Geometry: final body of the model. Coordinates: model frame, mm. A direction names the side the tool comes from. Coordinates: 2 decimals unless noted, no trailing zeros. Write each loop counter-clockwise with the first axis right and the second up, starting at its lowest first coordinate (ties: lowest second). Pieces come first, ordered by that corner, then holes. Notation, with made-up numbers: (63.5, 14) -> (105.5, 14) arc R15 cw to (105.5, 29) -> close; hole circle Ø9 at (71, -33). An arc over 180 degrees is marked (long way). One line per item, written item: value.
```python
from build123d import *

# Parameters (mm, degrees)
SCHIZZO2_R                   = 5.1
SCHIZZO2_R_2                 = 3.5
ESTRUSIONE_ESTRUSIONE1_DEPTH = 8
SCHIZZO4_R                   = 11
TAGLIO_ESTRUSIONE1_DEPTH     = 3.7
SCHIZZO5_R                   = 1.1
TAGLIO_ESTRUSIONE2_DEPTH     = 3


with BuildPart() as part:
    # Schizzo2 → Estrusione-Estrusione1 (new body)
    with BuildSketch(Plane(origin=(0, 0, 0), x_dir=(1, 0, 0), z_dir=(0, 1, 0))):
        with BuildLine():
            Line((70, -15), (-70, -15))
            ThreePointArc((-70, -15), (-85, 0), (-70, 15))
            Line((-70, 15), (70, 15))
            ThreePointArc((70, 15), (85, 0), (70, -15))
        make_face()
        with Locations(Location((70, 0, 0), (0, 0, 270))):
            Circle(SCHIZZO2_R, mode=Mode.SUBTRACT)
        with Locations(Location((-70, 0, 0), (0, 0, 270))):
            Circle(SCHIZZO2_R_2, mode=Mode.SUBTRACT)
    extrude(amount=ESTRUSIONE_ESTRUSIONE1_DEPTH)

    # Schizzo4 → Taglio-Estrusione1 (cut)
    with BuildSketch(Plane.XZ):
        with Locations(Location((-70, 0, 0), (0, 0, 270))):
            Circle(SCHIZZO4_R)
    extrude(amount=-TAGLIO_ESTRUSIONE1_DEPTH, mode=Mode.SUBTRACT)

    # Schizzo5 → Taglio-Estrusione2 (cut)
    with BuildSketch(Plane.XZ.offset(-3.7)):
        with Locations(Location((-75.66, 5.66, 0), (0, 0, 270))):
            Circle(SCHIZZO5_R)
        with Locations(Location((-64.34, 5.66, 0), (0, 0, 90))):
            Circle(SCHIZZO5_R)
        with Locations(Location((-64.34, -5.66, 0), (0, 0, 270))):
            Circle(SCHIZZO5_R)
        with Locations(Location((-75.66, -5.66, 0), (0, 0, 90))):
            Circle(SCHIZZO5_R)
    extrude(amount=-TAGLIO_ESTRUSIONE2_DEPTH, mode=Mode.SUBTRACT)


solid = part.part
```
(1) Section D-D (z = 8.5). Return the cut outline in (x, y), then the cut area to 3 significant figures.
Responses:
outline: (-82.36, 0) -> (-76.98, 0) -> (-76.98, 3.7) -> (-63.02, 3.7) -> (-63.02, 0) -> (82.36, 0) -> (82.36, 8) -> (-82.36, 8) -> close
area: 1,270 mm2
(2) Line query: line 1 (X direction, y = 4.7, z = 0); line 2 (Z direction, x = -64.34, y = 4.4); line 3 (X direction, y = 4.75, z = 5.66). Output: solid intervals per line, ascending. Write a range as [from, to].
Responses:
line 1: x = [-85, -73.5], [-66.5, 64.9], [75.1, 85]
line 2: z = [-15, -6.76], [-4.56, 4.56], [6.76, 15]
line 3: x = [-83.89, -76.76], [-74.56, -65.44], [-63.24, 83.89]
(3) Pull-direction query (Z, two-part tool) for faces 3 (the cylindrical face through (-59.094, 1.824, 1.432)), 4 (the flat face through (1, 4, 15)), 5 (the flat face through (1, 0, 0)); classes: released by +Z, released by -Z, zero draft, split by the parting line, or undercut.
Responses:
face 3: undercut
face 4: released by +Z
face 5: zero draft
(4) Section A-A (x = 72). Return the cut outline in (y, z).
Responses:
outline: (0, -14.87) -> (8, -14.87) -> (8, -4.69) -> (0, -4.69) -> close; (0, 4.69) -> (8, 4.69) -> (8, 14.87) -> (0, 14.87) -> close
(5) Reachability of faces 1 (the cylindrical face through (75, 4, -1)), 2 (the flat face through (-67, 3.7, 3)) from +Z, -Z, +X, -X, +Y, -Y: full face, straight path, thin tool, end or side. Return the list, or none.
Responses:
face 1: +Y, -Y
face 2: -Y
(6) First-contact query: pin 1 (17.5 mm diameter, centred on x = -70, z = 0, fed in from -Y); pin 2 (11 mm diameter, centred on x = -70, z = 0, fed in from +Y); pin 3 (1.3 mm diameter, centred on x = -64.34, z = -5.66, fed in from -Y); pin 4 (9 mm diameter, centred on x = 70, z = 0, fed in from -Y). Flat tips, straight axial feed; report the tip coordinate or a pass-through.
Responses:
pin 1: stops at y = 3.7
pin 2: stops at y = 8
pin 3: stops at y = 6.7
pin 4: passes through
(7) Section C-C (z = -0.5). Return the cut outline in (x, y).
Responses:
outline: (-84.99, 0) -> (-80.99, 0) -> (-80.99, 3.7) -> (-73.46, 3.7) -> (-73.46, 8) -> (-84.99, 8) -> close; (-66.54, 3.7) -> (-59.01, 3.7) -> (-59.01, 0) -> (64.92, 0) -> (64.92, 8) -> (-66.54, 8) -> close; (75.08, 0) -> (84.99, 0) -> (84.99, 8) -> (75.08, 8) -> close
(8) Section B-B (y = 1.5). Return the cut outline in (x, z).
Responses:
outline: (-70, -15) -> (70, -15) arc R15 ccw to (70, 15) -> (-70, 15) arc R15 ccw to start; hole circle Ø22 at (-70, 0); hole circle Ø10.2 at (70, 0)
